Geometry: final body of the model. Coordinates: model frame, mm. A direction names the side the tool comes from. Give positions to 0.01 mm unless a question says otherwise; leave off trailing zeros. Write each loop counter-clockwise with the first axis right and the second up, starting at its lowest first coordinate (ties: lowest second). Pieces come first, ordered by that corner, then holes.
Q1. Pin query (flat end, axial travel): pin 1 (16.5 mm diameter, centred on x = -7.5, y = -3, fed in from +Z); pin 2 (10 mm diameter, centred on x = 4.5, z = 1.5, fed in from -Y); pin 3 (1.5 mm diameter, centred on x = -0.5, y = 0, fed in from -Z). Return the tip coordinate at first contact, or that it passes through.
Q2. Line query: L1, parallel to X at y = 12, z = 12.5; L2, parallel to Z at x = -7, y = -27; L3, parallel to X at y = -21.5, z = -17. Output: solid intervals per line, ascending.
Q3. Cut plane B-B on x = 0. Return the cut outline in (y, z).
Q4. Cut plane C-C on y = -3.5. Return the cut outline in (x, z).
Q5. Cut plane A-A on z = -9. Return the cut outline in (x, y), plus the area to 3 significant figures.
Q6. Reachability of faces 1 (the face through (-0.54, 2.44, -26.39)), 2 (the face through (-20.059, 22.896, 5.722)), 3 (the face through (0, 28, 26.883)) from +Z, -Z, +X, -X, +Y, -Y: full face, straight path, thin tool, end or side. Return the list, or none.
Q7. Cut plane D-D on x = 12. Return the cut outline in (y, z).
Q8. Draft query along X for faces 4 (the face through (0, 0, -25.883)), 5 (the face through (20.059, 22.896, 5.722)), 6 (the face through (-28.915, 31.799, 4.639)), 7 (the face through (0, 32.4, 1)). Return one class per face: pulls with the +X half, pulls with the -X half, needs draft (parallel to the pull), parting line crosses it, or undercut.
```python
from build123d import *

# Parameters (mm, degrees)
F0_W     = 58.9698813856
F0_H     = 53.7666678429
F1_DEPTH = 32.4
F2_T     = -8
F3_R     = 5
F4_R     = 10.8639610307
F5_R     = 2
F6_R     = 1
F7_R     = 2.5
F8_DEPTH = 1


with BuildPart() as f1:
    # F0 (on Front) → F1 (new body, symmetric)
    with BuildSketch(Plane.XZ):
        Rectangle(F0_W, F0_H)
    extrude(amount=F1_DEPTH, both=True)

    # F2
    f2_openings = [f1.faces().sort_by_distance(p)[0] for p in [
        (0, 0, 26.883334),
        (0, -32.4, 0),
    ]]
    offset(amount=F2_T, openings=f2_openings)

    # F3
    f3_edges = [f1.edges().sort_by_distance(p)[0] for p in [
        (0, 24.4, -18.883334),
        (0, -32.4, -18.883334),
        (-21.484941, -4, -18.883334),
        (21.484941, -4, -18.883334),
        (-21.484941, 24.4, 4),
        (21.484941, 24.4, 4),
        (21.484941, -32.4, 4),
        (-21.484941, -32.4, 4),
    ]]
    fillet(f3_edges, radius=F3_R)

    # F4
    f4_edges = [f1.edges().sort_by_distance(p)[0] for p in [
        (29.484941, 0, -26.883334),
        (-29.484941, 0, -26.883334),
    ]]
    fillet(f4_edges, radius=F4_R)

    # F5
    f5_edges = [f1.edges().sort_by_distance(p)[0] for p in [
        (0, 32.4, -26.883334),
        (29.484941, 32.4, 5.431981),
        (26.30296, 32.4, -23.701353),
        (-26.30296, 32.4, -23.701353),
        (-29.484941, 32.4, 5.431981),
    ]]
    fillet(f5_edges, radius=F5_R)

    # F6
    f6_edges = [f1.edges().sort_by_distance(p)[0] for p in [
        (0, 24.4, 26.883334),
        (29.484941, -1, 26.883334),
        (28.899154, 31.814214, 26.883334),
        (27.984941, -32.4, 26.883334),
        (-27.984941, -32.4, 26.883334),
        (0, 32.4, 26.883334),
        (22.949407, -30.935534, 26.883334),
        (-28.899154, 31.814214, 26.883334),
        (21.484941, -4, 26.883334),
        (-29.484941, -1, 26.883334),
        (20.020475, 22.935534, 26.883334),
        (-22.949407, -30.935534, 26.883334),
        (-20.020475, 22.935534, 26.883334),
        (-21.484941, -4, 26.883334),
    ]]
    fillet(f6_edges, radius=F6_R)

    # F7 (on face) → F8 (cut)
    with BuildSketch(Plane(origin=(0, 0, -26.8833339214), x_dir=(1, 0, 0), z_dir=(0, 0, -1))):
        Circle(F7_R)
    extrude(amount=-F8_DEPTH, mode=Mode.SUBTRACT)


solid = f1.part
```
Data:
1. pin 1: stops at z = -18.88
1. pin 2: stops at y = 24.4
1. pin 3: stops at z = -25.88
2. L1: x = -29.48 to -21.48, 21.48 to 29.48
2. L2: z = -26.88 to -18.88
2. L3: x = -29.44 to -20.39, 20.39 to 29.44
3. outline: (-32.4, -26.88) - (-2.5, -26.88) - (-2.5, -25.88) - (2.5, -25.88) - (2.5, -26.88) - (30.4, -26.88) arc R2 ccw to (32.4, -24.88) - (32.4, 25.88) arc R1 ccw to (31.4, 26.88) - (25.4, 26.88) arc R1 ccw to (24.4, 25.88) - (24.4, -13.88) arc R5 cw to (19.4, -18.88) - (-27.4, -18.88) arc R5 ccw to (-32.4, -23.88) - close
4. outline: (-29.48, -16.02) arc R10.86 ccw to (-18.62, -26.88) - (18.62, -26.88) arc R10.86 ccw to (29.48, -16.02) - (29.48, 25.88) arc R1 ccw to (28.48, 26.88) - (22.48, 26.88) arc R1 ccw to (21.48, 25.88) - (21.48, -13.88) arc R5 cw to (16.48, -18.88) - (-16.48, -18.88) arc R5 cw to (-21.48, -13.88) - (-21.48, 25.88) arc R1 ccw to (-22.48, 26.88) - (-28.48, 26.88) arc R1 ccw to (-29.48, 25.88) - close
5. outline: (-29.48, -32.4) - (-26.48, -32.4) arc R5 ccw to (-21.48, -27.4) - (-21.48, 19.4) arc R5 cw to (-16.48, 24.4) - (16.48, 24.4) arc R5 cw to (21.48, 19.4) - (21.48, -27.4) arc R5 ccw to (26.48, -32.4) - (29.48, -32.4) - (29.48, 30.4) arc R2 ccw to (27.48, 32.4) - (-27.48, 32.4) arc R2 ccw to (-29.48, 30.4) - close
5. area: 1,380 mm2
6. face 1: -Z
6. face 2: +Z, -Y
6. face 3: +Z, +X, -X, +Y, -Y
7. outline: (-32.4, -26.88) - (30.4, -26.88) arc R2 ccw to (32.4, -24.88) - (32.4, 25.88) arc R1 ccw to (31.4, 26.88) - (25.4, 26.88) arc R1 ccw to (24.4, 25.88) - (24.4, -13.88) arc R5 cw to (19.4, -18.88) - (-27.4, -18.88) arc R5 ccw to (-32.4, -23.88) - close
8. face 4: undercut
8. face 5: undercut
8. face 6: pulls with the -X half
8. face 7: needs draft
